Geometry check sheet. Reference: the model listing, model coordinates, mm. A direction names the side the tool comes from. Coordinates: 2 decimals unless noted, no trailing zeros. Loops run counter-clockwise (first coordinate to the right, second up) from the corner with the lowest first, then second, coordinate; pieces in that order, holes last. Notation, with made-up numbers: (29, 73.5) - (67, 73.5) arc R14 cw to (67, 89.5) - close; hole circle Ø2 at (42, -23). An arc over 180 degrees is marked (long way). Write item = value, one per line. Start each with the question number.
from build123d import *

# Parameters (mm, degrees)
SKETCH1_W           = 90.8
SKETCH1_H           = 100
BOSS_EXTRUDE1_DEPTH = 62.8
CUT_EXTRUDE2_DEPTH  = 50
SKETCH3_R           = 3.25
BOSS_EXTRUDE2_DEPTH = 1.8
FILLET3_R           = 1.8
SKETCH4_R           = 2.25
BOSS_EXTRUDE3_DEPTH = 0.5
SKETCH6_R           = 6.75
BOSS_EXTRUDE4_DEPTH = 2.2
CHAMFER2_SIZE       = 1.4


with BuildPart() as part:
    # Sketch1 → Boss-Extrude1 (new body)
    with BuildSketch(Plane(origin=(0, 0, 0), x_dir=(1, 0, 0), z_dir=(0, 1, 0))):
        Rectangle(SKETCH1_W, SKETCH1_H)
    extrude(amount=BOSS_EXTRUDE1_DEPTH)

    # Sketch2 → Cut-Extrude2 (cut)
    with BuildSketch(Plane(origin=(0, 0, 0), x_dir=(-1, 0, 0), z_dir=(0, -1, 0))):
        with BuildLine():
            Line((33.550736089, -1.55), (33.550736089, -5.448527997))
            ThreePointArc((33.550736089, -5.448527997), (31.999263911, -7.000000175), (30.447791734, -5.448527997))
            Line((30.447791734, -5.448527997), (30.447791734, -1.55))
            Line((30.447791734, -1.55), (26.55, -1.55))
            ThreePointArc((26.55, -1.55), (25, 0), (26.55, 1.55))
            Line((26.55, 1.55), (30.447791734, 1.55))
            Line((30.447791734, 1.55), (30.447791734, 5.448527997))
            ThreePointArc((30.447791734, 5.448527997), (31.999263911, 7.000000175), (33.550736089, 5.448527997))
            Line((33.550736089, 5.448527997), (33.550736089, 1.55))
            Line((33.550736089, 1.55), (37.45, 1.55))
            ThreePointArc((37.45, 1.55), (39, 0), (37.45, -1.55))
            Line((37.45, -1.55), (33.550736089, -1.55))
        make_face()
        with BuildLine():
            Line((-30.447791734, 1.55), (-30.447791734, 5.448527997))
            ThreePointArc((-30.447791734, 5.448527997), (-31.999263911, 7.000000175), (-33.550736089, 5.448527997))
            Line((-33.550736089, 5.448527997), (-33.550736089, 1.55))
            Line((-33.550736089, 1.55), (-37.45, 1.55))
            ThreePointArc((-37.45, 1.55), (-39, 0), (-37.45, -1.55))
            Line((-37.45, -1.55), (-33.550736089, -1.55))
            Line((-33.550736089, -1.55), (-33.550736089, -5.448527997))
            ThreePointArc((-33.550736089, -5.448527997), (-31.999263911, -7.000000175), (-30.447791734, -5.448527997))
            Line((-30.447791734, -5.448527997), (-30.447791734, -1.55))
            Line((-30.447791734, -1.55), (-26.55, -1.55))
            ThreePointArc((-26.55, -1.55), (-25, 0), (-26.55, 1.55))
            Line((-26.55, 1.55), (-30.447791734, 1.55))
        make_face()
    extrude(amount=-CUT_EXTRUDE2_DEPTH, mode=Mode.SUBTRACT)

    # Sketch3 → Boss-Extrude2 (add)
    with BuildSketch(Plane.XZ):
        with Locations(Location((31.999263911, 35.350000175, 0), (0, 0, 270))):
            Circle(SKETCH3_R)
        with Locations(Location((31.999263911, -35.350000175, 0), (0, 0, 270))):
            Circle(SKETCH3_R)
        with Locations(Location((-31.999263911, -35.350000175, 0), (0, 0, 90))):
            Circle(SKETCH3_R)
        with Locations(Location((-31.999263911, 35.350000175, 0), (0, 0, 90))):
            Circle(SKETCH3_R)
    extrude(amount=BOSS_EXTRUDE2_DEPTH)

    # Fillet3
    fillet3_edges = [part.edges().sort_by_distance(p)[0] for p in [
        (-31.999263911, -1.8, 32.100000175),
        (31.999263911, -1.8, -32.100000175),
        (31.999263911, -1.8, 38.600000175),
        (-31.999263911, -1.8, -38.600000175),
    ]]
    fillet(fillet3_edges, radius=FILLET3_R - 0.0001)  # a hair under: the kernel refuses the full size

    # Sketch4 → Boss-Extrude3 (add)
    with BuildSketch(Plane(origin=(0, 0, 0), x_dir=(-1, 0, 0), z_dir=(0, -1, 0))):
        with Locations(Location((18.65, -44.25, 0), (0, 0, 90))):
            Circle(SKETCH4_R)
        with Locations(Location((-39.15, -44.25, 0), (0, 0, 90))):
            Circle(SKETCH4_R)
        with Locations(Location((-39.15, 44.25, 0), (0, 0, 270))):
            Circle(SKETCH4_R)
        with Locations(Location((18.65, 44.25, 0), (0, 0, 270))):
            Circle(SKETCH4_R)
    extrude(amount=BOSS_EXTRUDE3_DEPTH)

    # Sketch6 → Boss-Extrude4 (add)
    with BuildSketch(Plane.ZY.offset(45.4)):
        with Locations(Location((24.75, 49.55, 0), (0, 0, 180))):
            Circle(SKETCH6_R)
    extrude(amount=BOSS_EXTRUDE4_DEPTH)

    # Chamfer2
    chamfer2_edges = [part.edges().sort_by_distance(p)[0] for p in [
        (-47.6, 49.55, 31.5),
    ]]
    chamfer(chamfer2_edges, length=CHAMFER2_SIZE)


solid = part.part
(1) Sectioned sample at D-D on x = 11. Enter the section's corners in (y, z).
(2) Tool access check on faces 1 (the face through (-39, 25, 0)), 2 (the face through (39, -0.5, 44)). Record the directions out of +Z, -Z, +X, -X, +Y, -Y that give a thin tool (end or side, any length) a straight path to the whole face; none if there is none.
(3) Scan lines: line 1 (Z direction, x = 37.5, y = 22); line 2 (Z direction, x = 32, y = 45); line 3 (Y direction, x = 21, z = -38). Record each from-to range of solid material in increasing order.
(4) Draft check along X on faces 3 (the face through (25, 25, 0)), 4 (the face through (32, 50, 0)), 5 (the face through (-47.6, 49, 25)), 6 (the face through (39, -0.5, -44)). Enter one of: pulls with the +X half, pulls with the -X half, needs draft (parallel to the pull), parting line crosses it, or undercut.
(5) Sectioned sample at A-A on y = 5.5. Enter the section's corners in (x, z).
(6) Sectioned sample at B-B on z = 24.75. Enter the section's corners in (x, y).
(7) Sectioned sample at C-C on z = -44.25. Enter the section's corners in (x, y).
(8) Depth check by flat-ended pin: pin 1 (7 mm diameter, centred on x = 33, z = 1, fed in from -Y); pin 2 (1.3 mm diameter, centred on x = 39.5, z = -45.5, fed in from -Y); pin 3 (1.5 mm diameter, centred on y = 45, z = 12.5, fed in from -X). Enter the tip coordinate at first touch or a pass-through.
Working result:
q1.outline = (0, -50) - (62.8, -50) - (62.8, 50) - (0, 50) - close
q2.face_1 = -Y
q2.face_2 = +Z, -Z, +X, -X, -Y
q3.line_1 = -50 to -1.55, 1.55 to 50
q3.line_2 = -50 to -7, 7 to 50
q3.line_3 = 0 to 62.8
q4.face_3 = undercut
q4.face_4 = undercut
q4.face_5 = pulls with the -X half
q4.face_6 = needs draft
q5.outline = (-45.4, -50) - (45.4, -50) - (45.4, 50) - (-45.4, 50) - close; hole (-37.45, -1.55) - (-33.55, -1.55) - (-33.55, -5.45) arc R1.55 ccw to (-30.45, -5.45) - (-30.45, -1.55) - (-26.55, -1.55) arc R1.55 ccw to (-26.55, 1.55) - (-30.45, 1.55) - (-30.45, 5.45) arc R1.55 ccw to (-33.55, 5.45) - (-33.55, 1.55) - (-37.45, 1.55) arc R1.55 ccw to start; hole (26.55, -1.55) - (30.45, -1.55) - (30.45, -5.45) arc R1.55 ccw to (33.55, -5.45) - (33.55, -1.55) - (37.45, -1.55) arc R1.55 ccw to (37.45, 1.55) - (33.55, 1.55) - (33.55, 5.45) arc R1.55 ccw to (30.45, 5.45) - (30.45, 1.55) - (26.55, 1.55) arc R1.55 ccw to start
q6.outline = (-47.6, 44.2) - (-46.2, 42.8) - (-45.4, 42.8) - (-45.4, 0) - (45.4, 0) - (45.4, 62.8) - (-45.4, 62.8) - (-45.4, 56.3) - (-46.2, 56.3) - (-47.6, 54.9) - close
q7.outline = (-45.4, 0) - (-20.9, 0) - (-20.9, -0.5) - (-16.4, -0.5) - (-16.4, 0) - (36.9, 0) - (36.9, -0.5) - (41.4, -0.5) - (41.4, 0) - (45.4, 0) - (45.4, 62.8) - (-45.4, 62.8) - close
q8.pin_1 = 0
q8.pin_2 = -0.5
q8.pin_3 = -45.4
